Design review of the part built by this model. Coordinates are the model's own, in mm. Face numbers are marked on the shaded views. A direction names the side the tool comes from. Coordinates: 2 decimals unless noted, no trailing zeros. Write each loop counter-clockwise with the first axis right and the second up, starting at its lowest first coordinate (ties: lowest second). Pieces come first, ordered by that corner, then holes. Notation, with made-up numbers: (46, -36) -> (99, -36) arc R27 cw to (99, -9) -> close; hole circle Ø11 at (54.5, 67.25). An arc over 180 degrees is marked (long way). Answer in a Markdown table with one row per item. Add a question column.
Item 1: Draft analysis for pull direction Y (two halves, no side actions). For the marked faces 4, 5, 6 and 7, state which applies: released by +Y, released by -Y, zero draft, split by the parting line, or undercut.
Item 2: Clearance check with flat-ended pins moving along their axes: P1, Ø0.5, axis at y = 12.5, z = 2, coming from the -X side; P2, Ø0.8, axis at y = -12, z = 2, coming from the +X side. State where each tip first meets the part, or that it passes through.
Item 3: For the marked faces 1, 2 and 3, list the 3-axis set-ups (+Z, -Z, +X, -X, +Y, -Y) from which the entire face can be reached by the end or side of a thin tool; tool diameter is ignored.
Item 4: To check wall thickness, follow line 1 (Y direction, x = 13, z = 1.35); line 2 (X direction, y = 13, z = 2.05); line 3 (Y direction, x = -9.5, z = 0.6). State the ranges of each line that lie inside material, in increasing order.
Item 5: Take a section at A-A, the plane x = 9.5. Write out the cut boundary in (y, z), and give its area (3 significant figures).
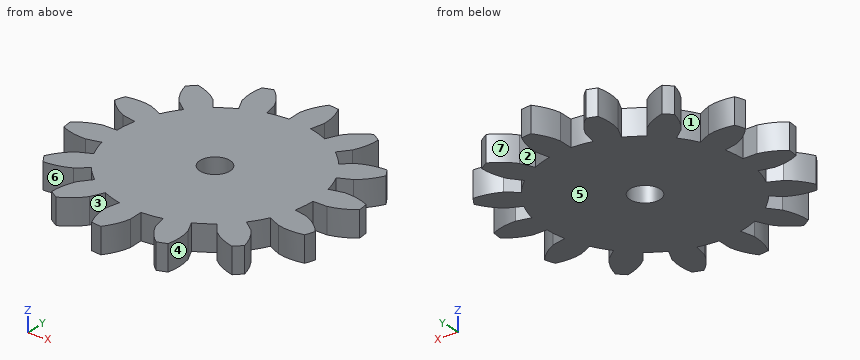
from build123d import *

# Parameters (mm, degrees)
BOSS_EXTRU_1_DEPTH           = 3
R_P_TITION_CIRCULAIRE2_COUNT = 14
ESQUISSE5_R                  = 11.5
BOSS_EXTRU_2_DEPTH           = 3
ESQUISSE6_R                  = 1.75
ENL_V_MAT_EXTRU_1_DEPTH      = 4


with BuildPart() as part:
    # Esquisse4 → Boss.-Extru.1 (new body)
    with BuildSketch(Plane.XY):
        with BuildLine():
            Line((0, 13.155696691), (0, 11.5))
            ThreePointArc((0, 11.5), (1.385979557, 11.416175396), (2.751754038, 11.165923594))
            Line((2.751754038, 11.165923594), (3.147934042, 12.773522094))
            ThreePointArc((3.147934042, 12.773522094), (3.010357566, 14.324173734), (2.517223611, 15.800746352))
            ThreePointArc((2.517223611, 15.800746352), (1.928319383, 15.883374464), (1.336751397, 15.944061456))
            ThreePointArc((1.336751397, 15.944061456), (0.504624377, 14.628382005), (0, 13.155696691))
        make_face()
    extrude(amount=BOSS_EXTRU_1_DEPTH)


with BuildPart() as r_p_tition_circulaire2_1:
    # R_p_tition circulaire2: pattern copy
    add(part.part.rotate(Axis((0, 0, 0), (0, 0, 1)), 1 * 360 / R_P_TITION_CIRCULAIRE2_COUNT))


with BuildPart() as r_p_tition_circulaire2_2:
    # R_p_tition circulaire2: pattern copy
    add(part.part.rotate(Axis((0, 0, 0), (0, 0, 1)), 2 * 360 / R_P_TITION_CIRCULAIRE2_COUNT))


with BuildPart() as r_p_tition_circulaire2_3:
    # R_p_tition circulaire2: pattern copy
    add(part.part.rotate(Axis((0, 0, 0), (0, 0, 1)), 3 * 360 / R_P_TITION_CIRCULAIRE2_COUNT))


with BuildPart() as r_p_tition_circulaire2_4:
    # R_p_tition circulaire2: pattern copy
    add(part.part.rotate(Axis((0, 0, 0), (0, 0, 1)), 4 * 360 / R_P_TITION_CIRCULAIRE2_COUNT))


with BuildPart() as r_p_tition_circulaire2_5:
    # R_p_tition circulaire2: pattern copy
    add(part.part.rotate(Axis((0, 0, 0), (0, 0, 1)), 5 * 360 / R_P_TITION_CIRCULAIRE2_COUNT))


with BuildPart() as r_p_tition_circulaire2_6:
    # R_p_tition circulaire2: pattern copy
    add(part.part.rotate(Axis((0, 0, 0), (0, 0, 1)), 6 * 360 / R_P_TITION_CIRCULAIRE2_COUNT))


with BuildPart() as r_p_tition_circulaire2_7:
    # R_p_tition circulaire2: pattern copy
    add(part.part.rotate(Axis((0, 0, 0), (0, 0, 1)), 7 * 360 / R_P_TITION_CIRCULAIRE2_COUNT))


with BuildPart() as r_p_tition_circulaire2_8:
    # R_p_tition circulaire2: pattern copy
    add(part.part.rotate(Axis((0, 0, 0), (0, 0, 1)), 8 * 360 / R_P_TITION_CIRCULAIRE2_COUNT))


with BuildPart() as r_p_tition_circulaire2_9:
    # R_p_tition circulaire2: pattern copy
    add(part.part.rotate(Axis((0, 0, 0), (0, 0, 1)), 9 * 360 / R_P_TITION_CIRCULAIRE2_COUNT))


with BuildPart() as r_p_tition_circulaire2_10:
    # R_p_tition circulaire2: pattern copy
    add(part.part.rotate(Axis((0, 0, 0), (0, 0, 1)), 10 * 360 / R_P_TITION_CIRCULAIRE2_COUNT))


with BuildPart() as r_p_tition_circulaire2_11:
    # R_p_tition circulaire2: pattern copy
    add(part.part.rotate(Axis((0, 0, 0), (0, 0, 1)), 11 * 360 / R_P_TITION_CIRCULAIRE2_COUNT))


with BuildPart() as r_p_tition_circulaire2_12:
    # R_p_tition circulaire2: pattern copy
    add(part.part.rotate(Axis((0, 0, 0), (0, 0, 1)), 12 * 360 / R_P_TITION_CIRCULAIRE2_COUNT))


with BuildPart() as r_p_tition_circulaire2_13:
    # R_p_tition circulaire2: pattern copy
    add(part.part.rotate(Axis((0, 0, 0), (0, 0, 1)), 13 * 360 / R_P_TITION_CIRCULAIRE2_COUNT))


with BuildPart() as part_1:
    add(part.part)

    add(r_p_tition_circulaire2_1.part)  # Boss.-Extru.2 merges R_p_tition circulaire2_1

    add(r_p_tition_circulaire2_2.part)  # Boss.-Extru.2 merges R_p_tition circulaire2_2

    add(r_p_tition_circulaire2_3.part)  # Boss.-Extru.2 merges R_p_tition circulaire2_3

    add(r_p_tition_circulaire2_4.part)  # Boss.-Extru.2 merges R_p_tition circulaire2_4

    add(r_p_tition_circulaire2_5.part)  # Boss.-Extru.2 merges R_p_tition circulaire2_5

    add(r_p_tition_circulaire2_6.part)  # Boss.-Extru.2 merges R_p_tition circulaire2_6

    add(r_p_tition_circulaire2_7.part)  # Boss.-Extru.2 merges R_p_tition circulaire2_7

    add(r_p_tition_circulaire2_8.part)  # Boss.-Extru.2 merges R_p_tition circulaire2_8

    add(r_p_tition_circulaire2_9.part)  # Boss.-Extru.2 merges R_p_tition circulaire2_9

    add(r_p_tition_circulaire2_10.part)  # Boss.-Extru.2 merges R_p_tition circulaire2_10

    add(r_p_tition_circulaire2_11.part)  # Boss.-Extru.2 merges R_p_tition circulaire2_11

    add(r_p_tition_circulaire2_12.part)  # Boss.-Extru.2 merges R_p_tition circulaire2_12

    add(r_p_tition_circulaire2_13.part)  # Boss.-Extru.2 merges R_p_tition circulaire2_13
    # Esquisse5 → Boss.-Extru.2 (add)
    with BuildSketch(Plane.XY):
        Circle(ESQUISSE5_R)
    extrude(amount=BOSS_EXTRU_2_DEPTH)

    # Esquisse6 → Enl_v. mat.-Extru.1 (cut, through all)
    with BuildSketch(Plane(origin=(0, 0, 0), x_dir=(-1, 0, 0), z_dir=(0, 0, -1))):
        Circle(ESQUISSE6_R)
    extrude(amount=-ENL_V_MAT_EXTRU_1_DEPTH, mode=Mode.SUBTRACT)


solid = part_1.part
Answers:
| question | item | result |
|---|---|---|
| 1 | face 4 | undercut |
| 1 | face 5 | zero draft |
| 1 | face 6 | released by -Y |
| 1 | face 7 | released by +Y |
| 2 | P1 | stops at x = -5.86 |
| 2 | P2 | stops at x = 11.02 |
| 3 | face 1 | +Z, -Z |
| 3 | face 2 | +Z, -Z, +Y |
| 3 | face 3 | +Z, -Z, -Y |
| 4 | line 1 | y = -6.11 to -3.01, -0.22 to 2.93, 6.49 to 8.89 |
| 4 | line 2 | x = -5.88 to -2.76, 0 to 3.15, 6.85 to 9.12 |
| 4 | line 3 | y = -7.58 to 6.48, 7.58 to 11.37 |
| 5 | outline | (-11.37, 0) -> (-7.58, 0) -> (-7.58, 3) -> (-11.37, 3) -> close; (-6.48, 0) -> (7.58, 0) -> (7.58, 3) -> (-6.48, 3) -> close |
| 5 | area | 53.6 mm^2 |
